from build123d import *

# Parameters (mm, degrees)
SKETCH2_W           = 48.5
SKETCH2_H           = 48.5
SKETCH2_R           = 15
SKETCH2_R_2         = 1.75
BOSS_EXTRUDE1_DEPTH = 3
SKETCH3_W           = 48.5
SKETCH3_H           = 48.5
SKETCH3_W_2         = 42.5
SKETCH3_H_2         = 42.5
BOSS_EXTRUDE2_DEPTH = 32
SKETCH4_W           = 68.5
SKETCH4_H           = 68.5
SKETCH4_R           = 1.75
SKETCH4_W_2         = 42.5
SKETCH4_H_2         = 42.5
BOSS_EXTRUDE3_DEPTH = 3
CHAMFER1_SIZE       = 15
SKETCH5_W           = 48.5
SKETCH5_H           = 48.5
SKETCH5_W_2         = 42.5
SKETCH5_H_2         = 42.5
BOSS_EXTRUDE4_DEPTH = 10
FILLET1_R           = 6
SKETCH7_W           = 45
SKETCH7_H           = 20
CUT_EXTRUDE2_DEPTH  = 20
FILLET2_R           = 4
CHAMFER2_SIZE       = 1.6
FILLET4_R           = 4
FILLET5_R           = 4
FILLET6_R           = 3


with BuildPart() as part:
    # Sketch2 → Boss-Extrude1 (new body)
    with BuildSketch(Plane(origin=(0, 0, 0), x_dir=(1, 0, 0), z_dir=(0, 1, 0))):
        Rectangle(SKETCH2_W, SKETCH2_H)
        Circle(SKETCH2_R, mode=Mode.SUBTRACT)
        with Locations((-15.5, 15.5)):
            Circle(SKETCH2_R_2, mode=Mode.SUBTRACT)
        with Locations((15.5, 15.5)):
            Circle(SKETCH2_R_2, mode=Mode.SUBTRACT)
        with Locations((15.5, -15.5)):
            Circle(SKETCH2_R_2, mode=Mode.SUBTRACT)
        with Locations((-15.5, -15.5)):
            Circle(SKETCH2_R_2, mode=Mode.SUBTRACT)
    extrude(amount=BOSS_EXTRUDE1_DEPTH)

    # Sketch3 → Boss-Extrude2 (add)
    with BuildSketch(Plane(origin=(0, 3, 0), x_dir=(1, 0, 0), z_dir=(0, 1, 0))):
        Rectangle(SKETCH3_W, SKETCH3_H)
        Rectangle(SKETCH3_W_2, SKETCH3_H_2, mode=Mode.SUBTRACT)
    extrude(amount=BOSS_EXTRUDE2_DEPTH)

    # Sketch4 → Boss-Extrude3 (add)
    with BuildSketch(Plane(origin=(0, 35, 0), x_dir=(1, 0, 0), z_dir=(0, 1, 0))):
        Rectangle(SKETCH4_W, SKETCH4_H)
        with Locations((-10, 30)):
            Circle(SKETCH4_R, mode=Mode.SUBTRACT)
        with Locations((10, 30)):
            Circle(SKETCH4_R, mode=Mode.SUBTRACT)
        with Locations((-29.25, 10)):
            Circle(SKETCH4_R, mode=Mode.SUBTRACT)
        with Locations((-29.25, -10)):
            Circle(SKETCH4_R, mode=Mode.SUBTRACT)
        with Locations((-10, -30)):
            Circle(SKETCH4_R, mode=Mode.SUBTRACT)
        with Locations((10, -30)):
            Circle(SKETCH4_R, mode=Mode.SUBTRACT)
        with Locations((29.25, -10)):
            Circle(SKETCH4_R, mode=Mode.SUBTRACT)
        with Locations((29.25, 10)):
            Circle(SKETCH4_R, mode=Mode.SUBTRACT)
        Rectangle(SKETCH4_W_2, SKETCH4_H_2, mode=Mode.SUBTRACT)
    extrude(amount=BOSS_EXTRUDE3_DEPTH)

    # Chamfer1
    chamfer1_edges = [part.edges().sort_by_distance(p)[0] for p in [
        (-34.25, 36.5, 34.25),
        (34.25, 36.5, 34.25),
        (34.25, 36.5, -34.25),
        (-34.25, 36.5, -34.25),
    ]]
    chamfer(chamfer1_edges, length=CHAMFER1_SIZE)

    # Sketch5 → Boss-Extrude4 (add)
    with BuildSketch(Plane.XZ):
        Rectangle(SKETCH5_W, SKETCH5_H)
        Rectangle(SKETCH5_W_2, SKETCH5_H_2, mode=Mode.SUBTRACT)
    extrude(amount=BOSS_EXTRUDE4_DEPTH)

    # Fillet1
    fillet1_edges = [part.edges().sort_by_distance(p)[0] for p in [
        (-24.25, 12.5, -24.25),
        (24.25, 12.5, -24.25),
        (24.25, 12.5, 24.25),
        (-24.25, 12.5, 24.25),
    ]]
    fillet(fillet1_edges, radius=FILLET1_R)

    # Sketch7 → Cut-Extrude2 (cut)
    with BuildSketch(Plane(origin=(24.25, 0, 0), x_dir=(0, 0, -1), z_dir=(1, 0, 0))):
        with Locations((14.25, 18)):
            Rectangle(SKETCH7_W, SKETCH7_H)
    extrude(amount=-CUT_EXTRUDE2_DEPTH, mode=Mode.SUBTRACT)

    # Fillet2
    fillet2_edges = [part.edges().sort_by_distance(p)[0] for p in [
        (-19.25, 36.5, 34.25),
        (19.25, 36.5, 34.25),
        (-19.25, 36.5, -34.25),
        (19.25, 36.5, -34.25),
        (-34.25, 36.5, 19.25),
        (-34.25, 36.5, -19.25),
        (34.25, 36.5, -19.25),
        (34.25, 36.5, 19.25),
    ]]
    fillet(fillet2_edges, radius=FILLET2_R)

    # Chamfer2
    chamfer2_edges = [part.edges().sort_by_distance(p)[0] for p in [
        (-17.25, 3, -15.5),
        (13.75, 3, -15.5),
        (13.75, 3, 15.5),
        (-17.25, 3, 15.5),
    ]]
    chamfer(chamfer2_edges, length=CHAMFER2_SIZE)

    # Fillet4
    fillet4_edges = [part.edges().sort_by_distance(p)[0] for p in [
        (21.25, 5.5, -21.25),
        (21.25, 33, -21.25),
        (-21.25, 20.5, -21.25),
        (-21.25, 20.5, 21.25),
        (21.25, 20.5, 21.25),
    ]]
    fillet(fillet4_edges, radius=FILLET4_R)

    # Fillet5
    fillet5_edges = [part.edges().sort_by_distance(p)[0] for p in [
        (4.25, 8, -22.75),
        (22.75, 28, 8.25),
        (4.25, 28, -22.75),
        (22.75, 8, 8.25),
    ]]
    fillet(fillet5_edges, radius=FILLET5_R)

    # Fillet6
    fillet6_edges = [part.edges().sort_by_distance(p)[0] for p in [
        (21.25, -5, 21.25),
        (-21.25, -5, 21.25),
        (-21.25, -5, -21.25),
        (21.25, -5, -21.25),
    ]]
    fillet(fillet6_edges, radius=FILLET6_R)


solid = part.part
Geometry check sheet. Reference: the model listing, model coordinates, mm. A direction names the side the tool comes from. Give positions to 0.01 mm unless a question says otherwise; leave off trailing zeros. Write each loop counter-clockwise with the first axis right and the second up, starting at its lowest first coordinate (ties: lowest second). Pieces come first, ordered by that corner, then holes.
1) Set-up check for faces 1 (the face through (-21.25, 20, 0)), 2 (the face through (22.539, 12.815, 22.446)), 3 (the face through (0, -5, 21.25)), 4 (the face through (22.729, 9.141, 7.047)), 5 (the face through (19.104, 36.521, 33.954)): record each of +Z, -Z, +X, -X, +Y, -Y from which the full face is reachable in a straight line by a thin tool's end or side.
Values follow:
face 1: +Y
face 2: +Z, +X, -Y
face 3: -Y
face 4: -Z, +X
face 5: +Z, +X, +Y, -Y
2) Go/stop test with flat-tipped pins: pin 1 Ø3 at (x, y) = (-22.5, 9) entering from +Z; pin 2 Ø5 at (x, y) = (13, 21) entering from +Z; pin 3 Ø4.5 at (x, z) = (29.25, -10) entering from -Y; pin 4 Ø5 at (x, z) = (-12.5, -20) entering from -Y. Record where each tip stops, or that it passes through.
Values follow:
pin 1: stops at z = 23.58
pin 2: stops at z = 24.25
pin 3: stops at y = 35
pin 4: stops at y = -10
3) Cross-section at A-A (x = 0). Record the boundary of the cut face in (y, z), plus the area to 4 significant figures.
Values follow:
outline: (-10, -24.25) - (35, -24.25) - (35, -34.25) - (38, -34.25) - (38, -21.25) - (3, -21.25) - (3, -15) - (0, -15) - (0, -21.25) - (-10, -21.25) - close; (-10, 21.25) - (0, 21.25) - (0, 15) - (3, 15) - (3, 21.25) - (38, 21.25) - (38, 34.25) - (35, 34.25) - (35, 24.25) - (-10, 24.25) - close
area: 385.5 mm2
4) Thickness scan on line 1 (Z direction, x = 10, y = 36.9); line 2 (X direction, y = 1.05, z = 15.5); line 3 (Z direction, x = 2, y = -8). Record the ranges inside material, lowest first.
Values follow:
line 1: z = -34.25 to -31.75, -28.25 to -21.25, 21.25 to 28.25, 31.75 to 34.25
line 2: x = -24.25 to -17.25, -13.75 to 13.75, 17.25 to 24.25
line 3: z = -24.25 to -21.25, 21.25 to 24.25
5) Cross-section at B-B (x = 29.25). Record the boundary of the cut face in (y, z).
Values follow:
outline: (35, -24.25) - (38, -24.25) - (38, -11.75) - (35, -11.75) - close; (35, -8.25) - (38, -8.25) - (38, 8.25) - (35, 8.25) - close; (35, 11.75) - (38, 11.75) - (38, 24.25) - (35, 24.25) - close
6) Cross-section at C-C (z = 30). Record the boundary of the cut face in (x, y).
Values follow:
outline: (-23.5, 35) - (-11.75, 35) - (-11.75, 38) - (-23.5, 38) - close; (-8.25, 35) - (8.25, 35) - (8.25, 38) - (-8.25, 38) - close; (11.75, 35) - (23.5, 35) - (23.5, 38) - (11.75, 38) - close
7) Cross-section at D-D (z = -10). Count the separate pieces of the cut face and the enclosed holes in it, plus the area to 3 significant figures.
Values follow:
separate pieces: 5
enclosed holes: 0
area: 327 mm2
8) Release check for a two-part mould opening along X. For faces 6 (the face through (5.391, 26.797, -22.771)), 7 (the face through (-34.25, 36, 0)), 8 (the face through (0, -5, -21.25)) record: released by +X, released by -X, zero draft, split by the parting line, or undercut.
Values follow:
face 6: released by +X
face 7: released by -X
face 8: undercut
